```python
from build123d import *

# Parameters (mm, degrees)
F1_DEPTH = 3.175
F2_T     = -2.54
F3_D     = 1.27
F3_DEPTH = 3.176
F4_D     = 1.27


with BuildPart() as f1:
    # F0 (on Front) → F1 (new body, symmetric)
    with BuildSketch(Plane.XZ):
        Polygon((0, 46.7720143497), (0, 33.5211828351), (6.096, 33.5211828351), (9.144, 33.5211828351), (12.192, 33.5211828351), (24.384, 33.5211828351), (24.384, 46.7720143497), align=None)
    extrude(amount=F1_DEPTH, both=True)

    # F2
    f2_openings = [f1.faces().sort_by_distance(p)[0] for p in [
        (12.192, 0, 33.521183),
    ]]
    offset(amount=F2_T, openings=f2_openings)

    # F3 (through all, one way)
    with BuildSketch(Plane.XZ):
        with Locations((9.144, 37.4545268714)):
            Circle(F3_D / 2)
    extrude(amount=-F3_DEPTH, mode=Mode.SUBTRACT)

    # F4 (through all)
    with Locations(Plane(origin=(0, 0, 0), x_dir=(1, 0, 0), z_dir=(0, 1, 0))):
        with Locations((9.144, -37.4545268714)):
            Hole(F4_D / 2)


solid = f1.part
```
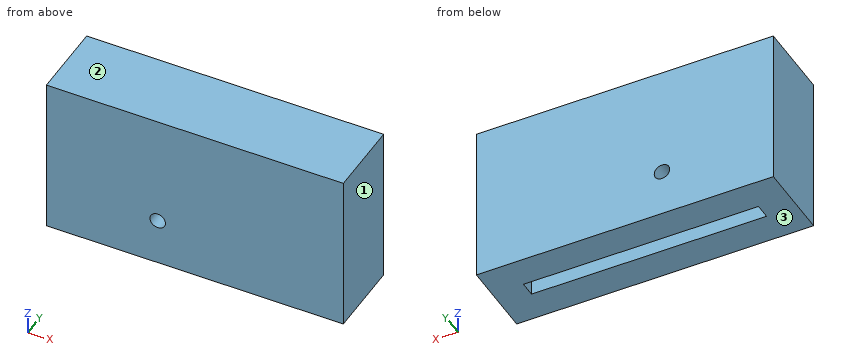
Check sheet for the modelled part. Datum: model origin and axes. Units: mm. Face numbers are marked on the shaded views. Round coordinates to 2 decimals unless told otherwise and drop trailing zeros. Loops run counter-clockwise (first coordinate to the right, second up) from the corner with the lowest first, then second, coordinate; pieces in that order, holes last. Notation, with made-up numbers: M -38.5,-18 L -25.5,-18 A28 cw -25.5,7 Z; hole C -26.5,4.25 d2. An arc over 180 degrees is marked long. Answer as a JSON object with one key per item and string values.
1. Section check B-B (x = 6.75). Record the boundary of the cut face in (y, z) (3 decimals).
Reply:
{"outline": "M -3.175,33.521 L -0.635,33.521 L -0.635,44.232 L 0.635,44.232 L 0.635,33.521 L 3.175,33.521 L 3.175,46.772 L -3.175,46.772 Z"}
2. Scan lines: line 1 (Y direction, x = 13.25, z = 39.25) (3 decimals); line 2 (X direction, y = 0, z = 40.75); line 3 (Z direction, x = 6.75, y = 0.5). Record each from-to range of solid material in increasing order.
Reply:
{"line 1": "y = -3.175 to -0.635, 0.635 to 3.175", "line 2": "x = 0 to 2.54, 21.84 to 24.38", "line 3": "z = 44.23 to 46.77"}
3. Mould release check, pull along Z, two halves, no side actions. Record for the marked faces 1, 2 and 3: pulls with the +Z half, pulls with the -Z half, needs draft (parallel to the pull), parting line crosses it, or undercut.
Reply:
{"face 1": "needs draft", "face 2": "pulls with the +Z half", "face 3": "pulls with the -Z half"}
4. Section check C-C (z = 43.5). Record the boundary of the cut face in (x, y) (3 decimals), plus the area to 3 significant figures.
Reply:
{"outline": "M 0,-3.175 L 24.384,-3.175 L 24.384,3.175 L 0,3.175 Z; hole M 2.54,-0.635 L 21.844,-0.635 L 21.844,0.635 L 2.54,0.635 Z", "area": "130 mm²"}
5. Section check D-D (z = 37.75). Record the boundary of the cut face in (x, y) (3 decimals), plus the area to 3 significant figures.
Reply:
{"outline": "M 0,-3.175 L 8.582,-3.175 L 8.582,-0.635 L 2.54,-0.635 L 2.54,0.635 L 8.582,0.635 L 8.582,3.175 L 0,3.175 Z; M 9.706,-3.175 L 24.384,-3.175 L 24.384,3.175 L 9.706,3.175 L 9.706,0.635 L 21.844,0.635 L 21.844,-0.635 L 9.706,-0.635 Z", "area": "125 mm²"}
6. Section check A-A (y = 0). Record the boundary of the cut face in (x, z), plus the area to 3 significant figures.
Reply:
{"outline": "M 0,33.52 L 2.54,33.52 L 2.54,44.23 L 21.84,44.23 L 21.84,33.52 L 24.38,33.52 L 24.38,46.77 L 0,46.77 Z", "area": "116 mm²"}
